Part model, mm, in its own coordinate system. Face numbers are marked on the shaded views. A direction names the side the tool comes from. Round coordinates to 2 decimals unless told otherwise and drop trailing zeros. Write each loop counter-clockwise with the first axis right and the second up, starting at its lowest first coordinate (ties: lowest second). Pieces come first, ordered by that corner, then holes.
1) Saw through at A-A on y = 2. Write the cut outline in (x, z), and give its area (3 significant figures).
2) Flat gauge pins, fed straight in: pin 1 (4 mm diameter, centred on y = -1.5, z = 4, fed in from +X); pin 2 (8 mm diameter, centred on x = 2.5, z = 18, fed in from +Y); pin 3 (5 mm diameter, centred on x = 3.5, z = 7, fed in from -Y); pin 4 (3 mm diameter, centred on x = 0.36, z = 5, fed in from +Y). Where does each tip first touch, or does it go through?
3) Pull direction Y, two halves, no side cores. Call the marked faces 1, 2, 3 and 4: +Y half, -Y half, draft (parallel to the pull), parting line (faces both ways), or undercut.
4) Saw through at D-D on z = 1.5. Write the cut outline in (x, y).
5) Saw through at C-C on x = -4.5. Write the cut outline in (y, z).
6) Which spindle directions (+Z, -Z, +X, -X, +Y, -Y) get a long thin tool onto all of the face, cutting with end or side? Do the marked faces 5, 6 and 7. Say none if no direction does.
7) Drill centre lines: L1, parallel to X at y = 4.5, z = 5; L2, parallel to Y at x = -3.75, z = 5; L3, parallel to Y at x = 2, z = 18.25. Where is each one in solid material? Low to high.
8) Saw through at B-B on z = 5. Write the cut outline in (x, y), and give its area (3 significant figures).
Autodesk Inventor part; units mm, degrees
ref_plane "YZ Plane" through (0, 0, 0) normal (1, 0, 0) x (0, 1, 0)
ref_plane "XZ Plane" through (0, 0, 0) normal (0, 1, 0) x (-1, 0, 0)
ref_plane "XY Plane" through (0, 0, 0) normal (0, 0, 1) x (1, 0, 0)
sketch "Эскиз1" plane through (0, 0, 0) normal (0, 0, 1) x (1, 0, 0)
  line L0 (7.5, -5) -> (7.5, 0)
  line L1 (5.0577, -5) -> (7.5, -5)
  line L2 (5.0577, -5) -> (-4.3392, -5)
  line L3 (-6.7815, -5) -> (-4.3392, -5)
  line L4 (-6.7815, -5) -> (-6.7815, 0)
  line L5 (-6.7815, 0) -> (-4.3392, 0)
  line L6 (5.0577, 0) -> (-4.3392, 0)
  line L7 (5.0577, 0) -> (7.5, 0)
  line L8 (7.5, -10.5) -> (-7.5, -10.5)
  line L9 (7.5, 0) -> (-6.7815, 0)
  line L10 (7.5, 10.5) -> (7.5, 0)
  line L11 (-7.5, 10.5) -> (7.5, 10.5)
  line L12 (-7.5, -10.5) -> (-7.5, 10.5)
  line L13 (7.5, -10.5) -> (-7.5, -10.5)
  line L14 (7.5, -5) -> (7.5, -10.5)
  line L15 (7.5, -5) -> (-6.7815, -5)
  line L16 (-6.7815, -5) -> (-6.7815, 0)
  point P0 (0, 0)
extrude "Выдавливание1" add sketch "Эскиз1" along normal blind 10 contours L14 L8 L12 L11 L10 L7 L6 L5 L4 L3 L2 L1
sketch "Эскиз2" plane through (-7.5, 10.5, 0) normal (0, 1, 0) x (1, 0, 0)
  circle A0 centre (7.8593, -5) radius 2
  point P0 (7.5, 0)
extrude "Выдавливание2" cut sketch "Эскиз2" against normal through all
sketch "Эскиз3" plane through (-7.5, 10.5, 0) normal (0, 1, 0) x (1, 0, 0)
  line L0 (15, -10) -> (0, -10)
  line L1 (15, -10) -> (15, -12.6449)
  line L2 (15, -12.6449) -> (0, -10)
  point P0 (7.5, 0)
  dimension "d5" = 10
extrude "Выдавливание3" add sketch "Эскиз3" against normal up to surface (21 mm away)
sketch "Эскиз4" plane through (7.5, -10.5, 12.6449) normal (-0.1736, 0, 0.9848) x (0.9848, 0, 0.1736)
  line L0 (-15.2314, 0) -> (0, 0)
  line L1 (0, 21) -> (0, 0)
  line L2 (-15.2314, 21) -> (0, 21)
  line L3 (-15.2314, 21) -> (-15.2314, 0)
  line L4 (-17.6157, -2.3843) -> (2.3843, -2.3843)
  line L5 (2.3843, -2.3843) -> (2.3843, 23.3843)
  line L6 (2.3843, 23.3843) -> (-17.6157, 23.3843)
  line L7 (-17.6157, 23.3843) -> (-17.6157, -2.3843)
  point P0 (-9.5818, 10.5)
  dimension "d8" = 20
extrude "Выдавливание4" add sketch "Эскиз4" along normal blind 2 contours L3 L2 L1 L0 | L7 L6 L5 L4
sketch "Эскиз5" plane through (7.1527, -10.5, 14.6145) normal (-0.1736, 0, 0.9848) x (0.9848, 0, 0.1736)
  line L0 (0.8843, 19) -> (-16.1157, 19)
  line L1 (-16.1157, 19) -> (-16.1157, 2)
  line L2 (-16.1157, 2) -> (0.8843, 2)
  line L3 (0.8843, 2) -> (0.8843, 19)
  line L4 (2.3843, -2.3843) -> (2.3843, 23.3843)
  line L5 (-17.6157, -2.3843) -> (2.3843, -2.3843)
  line L6 (-0.1157, 18) -> (-15.1157, 18)
  line L7 (-15.1157, 18) -> (-15.1157, 3)
  line L8 (-15.1157, 3) -> (-0.1157, 3)
  line L9 (-0.1157, 3) -> (-0.1157, 18)
  point P0 (-9.5818, 10.5)
  point P1 (0.8843, 10.5)
  point P2 (2.3843, 10.5)
  point P3 (-7.6157, 2)
  point P4 (-7.6157, -2.3843)
  dimension "d11" = 17
  dimension "d12" = 1
extrude "Выдавливание5" add sketch "Эскиз5" along normal blind 8
fillet "Сопряжение1" radius 2 8 edges at (7.329, -8.5, 18.7073) (7.329, 8.5, 18.7073) (-9.4128, 8.5, 15.7553) (-9.4128, -8.5, 15.7553) (-8.4279, 7.5, 15.9289) (6.3442, 7.5, 18.5337) (-8.4279, -7.5, 15.9289) (6.3442, -7.5, 18.5337)
equation "\"degg\" = 80deg"
properties part number "base_80"
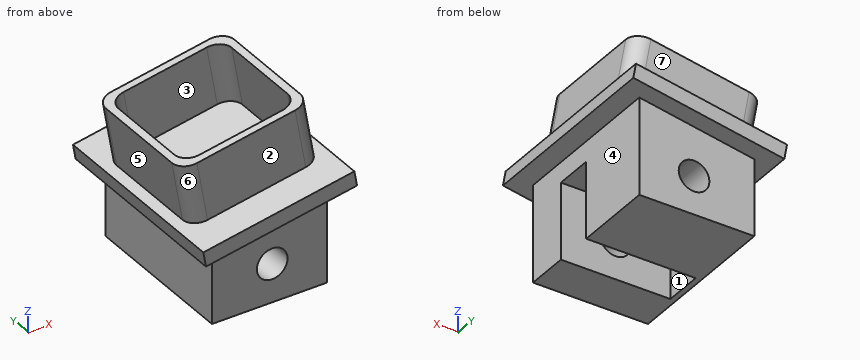
Completed:
1. outline: (-10.2, 11.56) - (-9.85, 9.59) - (-7.5, 10) - (-7.5, 0) - (7.5, 0) - (7.5, 12.64) - (9.85, 13.06) - (9.5, 15.03) - (8.02, 14.77) - (6.63, 22.65) - (5.65, 22.47) - (7.04, 14.59) - (-7.73, 11.99) - (-9.12, 19.87) - (-10.11, 19.69) - (-8.72, 11.82) - close; hole circle Ø4 at (0.36, 5)
1. area: 213 mm2
2. pin 1: stops at x = 7.5
2. pin 2: stops at y = 8.5
2. pin 3: stops at y = -10.5
2. pin 4: passes through
3. face 1: undercut
3. face 2: -Y half
3. face 3: undercut
3. face 4: draft
4. outline: (-7.5, -10.5) - (7.5, -10.5) - (7.5, -5) - (-6.78, -5) - (-6.78, 0) - (7.5, 0) - (7.5, 10.5) - (-7.5, 10.5) - close
5. outline: (-12.88, 10.53) - (-10.5, 10.53) - (-10.5, 0) - (-5, 0) - (-5, 10) - (0, 10) - (0, 0) - (10.5, 0) - (10.5, 10.53) - (12.88, 10.53) - (12.88, 12.56) - (8.5, 12.56) - (8.5, 20.68) - (7.5, 20.68) - (7.5, 12.56) - (-7.5, 12.56) - (-7.5, 20.68) - (-8.5, 20.68) - (-8.5, 12.56) - (-12.88, 12.56) - close
6. face 5: -X, +Y, -Y
6. face 6: -X, -Y
6. face 7: +Z, -X, +Y
7. L1: x = -7.5 to -1.64, 2.36 to 7.5
7. L2: y = -10.5 to -5, 0 to 10.5
7. L3: y = -8.5 to -7.5, 7.5 to 8.5
8. outline: (-7.5, -10.5) - (-1.64, -10.5) - (-1.64, -5) - (-6.78, -5) - (-6.78, 0) - (-1.64, 0) - (-1.64, 10.5) - (-7.5, 10.5) - close; (2.36, -10.5) - (7.5, -10.5) - (7.5, -5) - (2.36, -5) - close; (2.36, 0) - (7.5, 0) - (7.5, 10.5) - (2.36, 10.5) - close
8. area: 180 mm2
